```python
from build123d import *

# Parameters (mm, degrees)
F0_R      = 12.7
F1_DEPTH  = 2.54
F2_R      = 2.53999
F3_R      = 6.35
F4_DEPTH  = 0.635
F5_R      = 4.7625
F6_DEPTH  = 4.7244
F7_R      = 4.7625
F7_R_2    = 4.572
F8_DEPTH  = 4.7244
F9_R      = 4.572
F10_DEPTH = 1.778


# Not quite as in the source:
# - a fillet or chamfer is up to 0.001 mm smaller than in the source, because OpenCascade refuses the exact size


with BuildPart() as f1:
    # F0 (on Top) → F1 (new body)
    with BuildSketch(Plane.XY):
        Circle(F0_R)
    extrude(amount=F1_DEPTH)

    # F2 (radius 2.54 in the source; OpenCascade refuses exactly that, so slightly less here)
    f2_edges = [f1.edges().sort_by_distance(p)[0] for p in [
        (-12.7, 0, 0),
    ]]
    fillet(f2_edges, radius=F2_R)

    # F3 (on face) → F4 (join)
    with BuildSketch(Plane.XY.offset(2.54)):
        Circle(F3_R)
    extrude(amount=F4_DEPTH)

    # F5 (on face) → F6 (join)
    with BuildSketch(Plane.XY.offset(3.175)):
        Circle(F5_R)
    extrude(amount=F6_DEPTH)

    # F7 (on face) → F8 (cut, through all)
    with BuildSketch(Plane.XY.offset(7.8994)):
        Circle(F7_R)
        Circle(F7_R_2, mode=Mode.SUBTRACT)
    extrude(amount=-F8_DEPTH, mode=Mode.SUBTRACT)

    # F9 (on face) → F10 (cut)
    with BuildSketch(Plane.XY.offset(7.8994)):
        Circle(F9_R)
    extrude(amount=-F10_DEPTH, mode=Mode.SUBTRACT)


solid = f1.part
```
Part model, mm, in its own coordinate system. A direction names the side the tool comes from. Coordinates: 2 decimals unless noted, no trailing zeros. Write each loop counter-clockwise with the first axis right and the second up, starting at its lowest first coordinate (ties: lowest second). Pieces come first, ordered by that corner, then holes.
Item 1: Slice it at C-C (z = 5.25). Write the cut outline in (x, y).
Item 2: Probe line 1 (Z direction, x = 7.75, y = -3.25); line 2 (Z direction, x = 5, y = -3.25) (3 decimals); line 3 (X direction, y = 0.5, z = 5.5). List the from-to ranges inside material, lowest first.
Item 3: Slice it at D-D (z = 1.5). Write the cut outline in (x, y), and give its area (3 significant figures).
Item 4: Pin check, flat tips, straight feed: pin 1 (2 mm diameter, centred on x = -3.5, z = 4, fed in from +Y); pin 2 (1.5 mm diameter, centred on x = 8, y = 8, fed in from -Z); pin 3 (2 mm diameter, centred on x = -2.5, y = 9, fed in from +Z). Stop position of each tip, or through.
Item 5: Which spindle directions (+Z, -Z, +X, -X, +Y, -Y) get a long thin tool onto all of the face, cutting with end or side? Do faces 1 (the face through (0, 0, 0)), 2 (the face through (3, 6, 2.54)). Say none if no direction does.
Results found:
1. outline: circle Ø9.14 at (0, 0)
2. line 1: z = 0 to 2.54
2. line 2: z = 0 to 3.175
2. line 3: x = -4.54 to 4.54
3. outline: circle Ø24.95 at (0, 0)
3. area: 489 mm2
4. pin 1: stops at y = 5.63
4. pin 2: stops at z = 0.03
4. pin 3: stops at z = 2.54
5. face 1: -Z, +X, -X, +Y, -Y
5. face 2: +Z
